Study the drawing (mm; zero at the part's minimum x, y, z) and answer. Coordinates: 2 decimals unless noted, no trailing zeros. Order: outer loops, then holes, each group sorted by start corner. A loop starts at its lowest first (then second) coordinate and runs counter-clockwise, first axis right, second up. Notation, with made-up numbers: (-29.5, 64) -> (-25.5, 64) arc R13 ccw to (-25.5, 89) -> close; hole circle Ø9 at (-6, 73). An arc over 180 degrees is marked (long way). Answer as CSV lines item,"result". Start each with the question number.
Item 1: Straight lines are drawn through the part: L1, parallel to Y at x = 3.5, z = 2; L2, parallel to Y at x = 12.5, z = 4; L3, parallel to X at y = 8.5, z = 1.25 (1 decimal). For each, find the intervals that lie inside material, in ascending order.
Item 2: Section C-C (y = 11) is taken. Write down the section's boundary in (x, z), then the cut area to 3 significant figures.
Item 3: Section A-A (x = 3.5) is taken. Write down the section's boundary in (y, z).
Item 4: This flat-tipped pin is pushed along its axis until it touches: pin 1 Ø2 at (x, y) = (3.5, 7.5) entering from +Z. Where does it stop, or does it pass through?
Item 5: Section B-B (z = 4) is taken. Write down the section's boundary in (x, y), then the cut area to 3 significant figures.
Item 6: For a pull along Y with two mould halves and no side action, classify the marked faces 1, 2 and 3 as pulls with the +Y half, pulls with the -Y half, needs draft (parallel to the pull), parting line crosses it, or undercut.
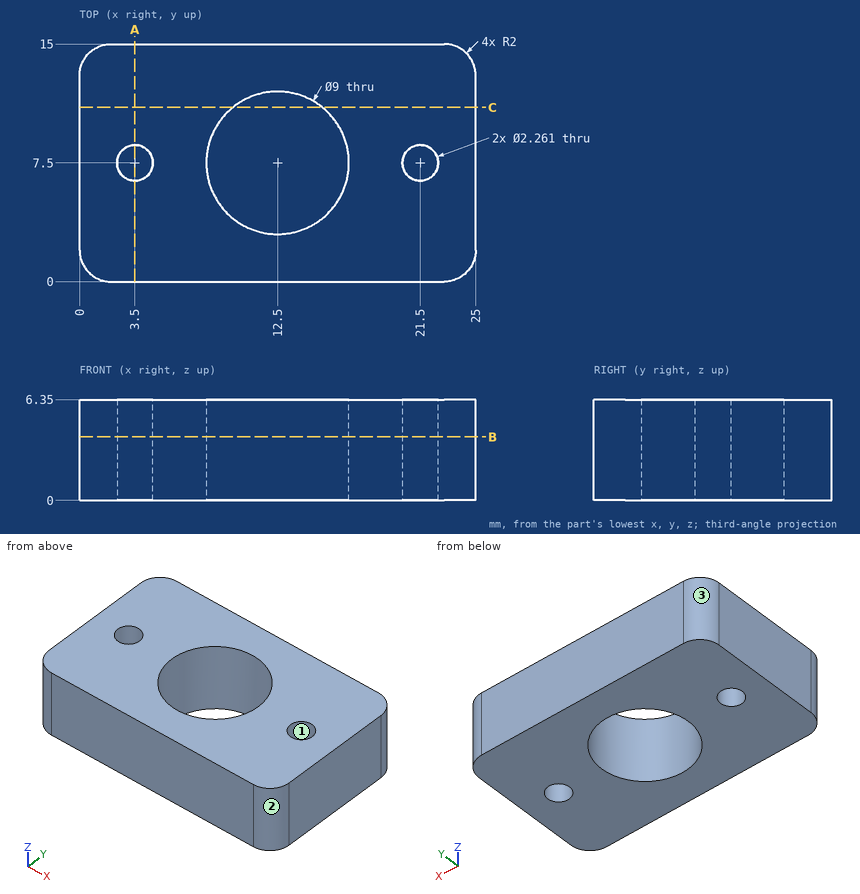
Checked values:
1,L1,"y = 0 to 6.37, 8.63 to 15"
1,L2,"y = 0 to 3, 12 to 15"
1,L3,"x = 0 to 3, 4 to 8.1, 16.9 to 21, 22 to 25"
2,outline,"(0, 0) -> (9.67, 0) -> (9.67, 6.35) -> (0, 6.35) -> close; (15.33, 0) -> (25, 0) -> (25, 6.35) -> (15.33, 6.35) -> close"
2,area,"123 mm^2"
3,outline,"(0, 0) -> (6.37, 0) -> (6.37, 6.35) -> (0, 6.35) -> close; (8.63, 0) -> (15, 0) -> (15, 6.35) -> (8.63, 6.35) -> close"
4,pin 1,"passes through"
5,outline,"(0, 2) arc R2 ccw to (2, 0) -> (23, 0) arc R2 ccw to (25, 2) -> (25, 13) arc R2 ccw to (23, 15) -> (2, 15) arc R2 ccw to (0, 13) -> close; hole circle Ø2.26 at (3.5, 7.5); hole circle Ø9 at (12.5, 7.5); hole circle Ø2.26 at (21.5, 7.5)"
5,area,"300 mm^2"
6,face 1,"undercut"
6,face 2,"pulls with the -Y half"
6,face 3,"pulls with the +Y half"
